Autodesk Inventor part; units mm, degrees
ref_plane "YZ Plane" through (0, 0, 0) normal (1, 0, 0) x (0, 1, 0)
ref_plane "XZ Plane" through (0, 0, 0) normal (0, 1, 0) x (-1, 0, 0)
ref_plane "XY Plane" through (0, 0, 0) normal (0, 0, 1) x (1, 0, 0)
sketch "Esquisse1" plane through (0, 0, 0) normal (0, 1, 0) x (-1, 0, 0)
  line L0 (18.0036, -31.6819) -> (18.0036, -41.5796)
  line L1 (18.0036, 33.4181) -> (18.0036, -31.6819)
  line L2 (18.0036, 33.4181) -> (18.0036, 41.5796)
  arc A0 (18.0036, -41.5796) -> (18.0036, 41.5796) centre (0, 0) ccw
  line L3 (21.0036, 36.7285) -> (21.0036, 33.4181)
  line L4 (21.0036, 33.4181) -> (21.0036, -31.6819)
  line L5 (21.0036, -31.6819) -> (21.0036, -36.7285)
  arc A1 (21.0036, -36.7285) -> (21.0036, 36.7285) centre (0, 0) ccw
  line L6 (45.0333, 5) -> (42.0135, 5)
  line L7 (42.0135, 5) -> (42.0135, -5)
  line L8 (42.0135, -5) -> (45.0333, -5)
  line L9 (45.0333, -5) -> (45.0333, 5)
  line L10 (45.0333, 5) -> (42.0135, -5) construction
  line L11 (42.0135, 5) -> (45.0333, -5) construction
  line L12 (49.818, 0) -> (34.3139, 0) construction
  point P0 (0, 0)
  point P1 (43.5234, 0)
  dimension "d7" = 90.62
  dimension "d8" = 3
  dimension "d9" = 10
extrude "Extrusion1" add sketch "Esquisse1" along normal blind 2 contours L8 A1 L6 L9 | L7 A1 | A1 L5 L4 L3 L7
fillet "Congé2" radius 3 2 edges at (-21.0036, 1, 36.7285) (-21.0036, 1, -36.7285)
sketch "Esquisse2" plane through (0, 2, 0) normal (0, 1, 0) x (1, 0, 0)
  point P0 (0, 0)
properties part number "Test_PCB"
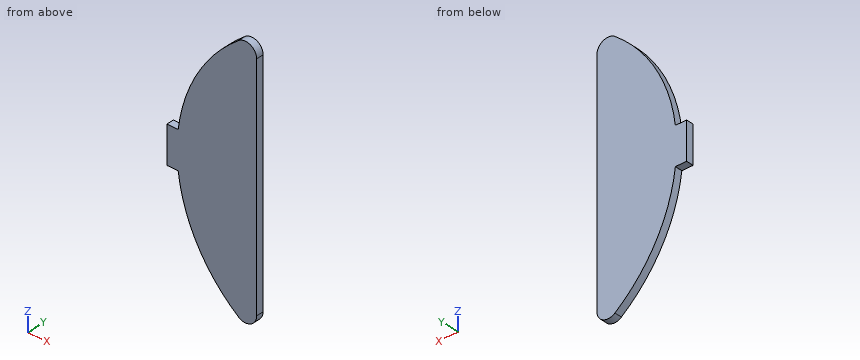
Part model, mm, in its own coordinate system. Round coordinates to 2 decimals unless told otherwise and drop trailing zeros. Write each loop counter-clockwise with the first axis right and the second up, starting at its lowest first coordinate (ties: lowest second). Pieces come first, ordered by that corner, then holes.
Item 1: Cut at B-B, the plane x = -34.5. Give the cut face in (y, z).
Results:
outline: (0, -24.49) - (2, -24.49) - (2, 24.49) - (0, 24.49) - close
Item 2: Probe L1, parallel to X at y = 0.2, z = 25; L2, parallel to Z at x = -44, y = 1.2; L3, parallel to Z at x = -26.75, y = 0.65. List the from-to ranges inside material, lowest first.
Results:
L1: x = -34.13 to -21
L2: z = -5 to 5
L3: z = -32.78 to 32.78
Item 3: Drop flat-ended pins along their axis: pin 1 Ø1 at (y, z) = (1, 19) entering from -X; pin 2 Ø0.6 at (x, y) = (-44, 0.5) entering from -Z; pin 3 Ø1 at (y, z) = (0.5, -11) entering from -X. Give the stop position or say it passes through.
Results:
pin 1: stops at x = -38.05
pin 2: stops at z = -5
pin 3: stops at x = -40.99
Item 4: Cut at A-A, the plane y = 0.4. Give the cut face in (x, z).
Results:
outline: (-45.03, -5) - (-42.01, -5) arc R42.31 ccw to (-25.84, -33.51) arc R3 ccw to (-21, -31.13) - (-21, 31.13) arc R3 ccw to (-25.84, 33.51) arc R42.31 ccw to (-42.01, 5) - (-45.03, 5) - close
Item 5: Cut at C-C, the plane z = 6.5. Give the cut face in (x, y), plus the area to 3 significant figures.
Results:
outline: (-41.81, 0) - (-21, 0) - (-21, 2) - (-41.81, 2) - close
area: 41.6 mm2
